from build123d import *

# Parameters (mm, degrees)
SKETCH1_W           = 10
SKETCH1_H           = 35
BOSS_EXTRUDE1_DEPTH = 5
SKETCH9_W           = 20
SKETCH9_H           = 11.5
BOSS_EXTRUDE3_DEPTH = 13
FILLET1_R           = 6
SKETCH10_W          = 15
SKETCH10_H          = 6.5
CUT_EXTRUDE4_DEPTH  = 17.5
CUT_EXTRUDE2_DEPTH  = 10
CHAMFER2_SIZE       = 6
CHAMFER2_SIZE_2     = 9.985676894


with BuildPart() as part:
    # Sketch1 → Boss-Extrude1 (new body)
    with BuildSketch(Plane.XY):
        with Locations((5, 17.5)):
            Rectangle(SKETCH1_W, SKETCH1_H)
    extrude(amount=BOSS_EXTRUDE1_DEPTH)

    # Sketch9 → Boss-Extrude3 (add)
    with BuildSketch(Plane.XZ):
        with Locations((0, 5.75)):
            Rectangle(SKETCH9_W, SKETCH9_H)
    extrude(amount=BOSS_EXTRUDE3_DEPTH)

    # Fillet1
    fillet1_edges = [part.edges().sort_by_distance(p)[0] for p in [
        (5, 0, 5),
    ]]
    fillet(fillet1_edges, radius=FILLET1_R)

    # Sketch10 → Cut-Extrude4 (cut)
    with BuildSketch(Plane.XZ.offset(13)):
        with Locations((0, 5.75)):
            Rectangle(SKETCH10_W, SKETCH10_H)
    extrude(amount=-CUT_EXTRUDE4_DEPTH, mode=Mode.SUBTRACT)

    # Sketch4 → Cut-Extrude2 (cut)
    with BuildSketch(Plane.XY.offset(5)):
        with BuildLine():
            Line((6.75, 32.5), (6.75, 7.5))
            ThreePointArc((6.75, 7.5), (5, 5.75), (3.25, 7.5))
            Line((3.25, 7.5), (3.25, 32.5))
            ThreePointArc((3.25, 32.5), (5, 34.25), (6.75, 32.5))
        make_face()
    extrude(amount=-CUT_EXTRUDE2_DEPTH, mode=Mode.SUBTRACT)

    # Chamfer2
    # the kernel refuses this chamfer: 9.985676894, 6 mm, written as the material it adds along each edge
    with BuildSketch(Plane(origin=(0, 0, 0), x_dir=(0.055087232083824676, 0.9984815455787568, 0), z_dir=(0, 0, 1))) as chamfer2_piece_1:
        Polygon((CHAMFER2_SIZE * 0.998481545579, CHAMFER2_SIZE * 0.0550872320838), (-CHAMFER2_SIZE_2 * 0.0550872320844, CHAMFER2_SIZE_2 * 0.998481545589), (0, 0), align=None)
    extrude(amount=2.5)
    with BuildSketch(Plane(origin=(0, 0, 0), x_dir=(0.055087232083824676, 0.9984815455787568, 0), z_dir=(0, 0, 1))) as chamfer2_piece_2_section:
        Polygon((CHAMFER2_SIZE * 0.998481545579, CHAMFER2_SIZE * 0.0550872320838), (-CHAMFER2_SIZE_2 * 0.0550872320844, CHAMFER2_SIZE_2 * 0.998481545589), (0, 0), align=None)
    chamfer2_piece_2 = extrude(amount=28.325253365, mode=Mode.PRIVATE)
    chamfer2_piece_2 = chamfer2_piece_2 - Plane(origin=(-0.832139741, 6, 11), x_dir=(0, 0, -1), z_dir=(-1, 0, 0)) * Cylinder(6, 97, mode=Mode.PRIVATE)
    chamfer2_piece_2 = split(chamfer2_piece_2, bisect_by=Plane(origin=(-0.832139741, 4.5, 3.75), z_dir=(0, 1, 0)), keep=Keep.TOP, mode=Mode.PRIVATE)
    chamfer2_piece_2 = split(chamfer2_piece_2, bisect_by=Plane(origin=(-0.832139741, 5, 11.5), z_dir=(0, 0, -1)), keep=Keep.TOP, mode=Mode.PRIVATE)
    add(chamfer2_piece_2)


solid = part.part
Can you work these out from the model? Positions are in its coordinate system, mm. A direction names the side the tool comes from. Coordinates: 2 decimals unless noted, no trailing zeros. Write each loop counter-clockwise with the first axis right and the second up, starting at its lowest first coordinate (ties: lowest second). Pieces come first, ordered by that corner, then holes.
Q1. Imagine slicing it at A-A, the plane z = 4.25. List the corners of the cut face in (x, y) for me, plus the area to 3 significant figures.
Results found:
outline: (-10, -13) - (-7.5, -13) - (-7.5, 0) - (-10, 0) - close; (-2.5, 4.5) - (7.5, 4.5) - (7.5, -13) - (10, -13) - (10, 35) - (0, 35) - (0, 6) - close; hole (3.25, 7.5) arc R1.75 ccw to (6.75, 7.5) - (6.75, 32.5) arc R1.75 ccw to (3.25, 32.5) - close
area: 286 mm2
Q2. Imagine slicing it at D-D, the plane y = -1.5. List the corners of the cut face in (x, z) for me.
Results found:
outline: (-10, 0) - (10, 0) - (10, 11.5) - (-10, 11.5) - close; hole (-7.5, 2.5) - (7.5, 2.5) - (7.5, 9) - (-7.5, 9) - close
Q3. If we mould it in two halves opening along X, with no side actions, what happens to faces 6 (the face through (10, 6, 4)), 7 (the face through (6.75, 20, 3)), 8 (the face through (0, 20, 2)), 9 (the face through (2, 0, 0))? For each: +X half, -X half, draft (parallel to the pull), parting line (faces both ways), or undercut.
Results found:
face 6: +X half
face 7: undercut
face 8: -X half
face 9: draft
Q4. Imagine slicing it at C-C, the plane x = 5. List the corners of the cut face in (y, z) for me, plus the area to 3 significant figures.
Results found:
outline: (-13, 0) - (5.75, 0) - (5.75, 5) - (6, 5) arc R6 cw to (4.5, 5.19) - (4.5, 2.5) - (-13, 2.5) - close; (-13, 9) - (0.34, 9) arc R6 cw to (0, 11) - (0, 11.5) - (-13, 11.5) - close; (34.25, 0) - (35, 0) - (35, 5) - (34.25, 5) - close
area: 86.6 mm2
Q5. For P1, Ø0.8, axis at x = 0.5, z = 3.5, coming from the -Y side; P2, Ø5, axis at x = 6.5, y = 25.5, coming from the +Z side; P3, Ø1.5, axis at y = 25, z = 2, coming from the -X side, each with a flat end and sliding along its axis, tell me the tip position at first contact or that it passes through.
Results found:
P1: stops at y = 4.5
P2: stops at z = 5
P3: stops at x = 0
Q6. Which directions (+Z, -Z, +X, -X, +Y, -Y) give clear straight access to the entire face, cutting with the end or side of a thin tool? Please do faces 1 (the face through (5.04, 5.75, 2.54)), 2 (the face through (7.5, -4, 6)), 3 (the face through (3, 21, 5)), 4 (the face through (3.25, 20, 3)), 5 (the face through (0, -6, 9)).
Results found:
face 1: -Z
face 2: -Y
face 3: +Z, +X, -X, +Y
face 4: +Z, -Z
face 5: +Y, -Y
Q7. Please list where these lines run through material, in increasing order: L1, parallel to X at y = 17, z = 1; L2, parallel to X at y = -4, z = 5.5; L3, parallel to Z at x = 1, y = -10.
Results found:
L1: x = 0 to 3.25, 6.75 to 10
L2: x = -10 to -7.5, 7.5 to 10
L3: z = 0 to 2.5, 9 to 11.5
Q8. Imagine slicing it at B-B, the plane y = 30. List the corners of the cut face in (x, z) for me, plus the area to 3 significant figures.
Results found:
outline: (0, 0) - (3.25, 0) - (3.25, 5) - (0, 5) - close; (6.75, 0) - (10, 0) - (10, 5) - (6.75, 5) - close
area: 32.5 mm2
